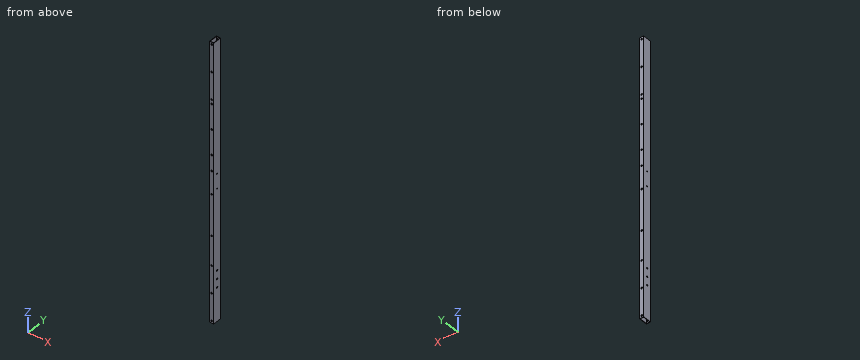
from build123d import *

# Parameters (mm, degrees)
SKETCH_1_W          = 10
SKETCH_1_H          = 20
SKETCH_1_W_2        = 7.6
SKETCH_1_H_2        = 17.6
EXTRUDE_1_DEPTH     = 660
SKETCH_2_R          = 2
CUT_EXTRUDE_1_DEPTH = 661.321891202
SKETCH_3_R          = 1.5
SKETCH_3_R_2        = 2
CUT_EXTRUDE_2_DEPTH = 661.151497764


with BuildPart() as part:
    # ｽｹｯﾁ1 → 押し出し-薄板1 (new body)
    with BuildSketch(Plane.XY):
        Rectangle(SKETCH_1_W, SKETCH_1_H)
        Rectangle(SKETCH_1_W_2, SKETCH_1_H_2, mode=Mode.SUBTRACT)
    extrude(amount=EXTRUDE_1_DEPTH)

    # ｽｹｯﾁ2 → ｶｯﾄ - 押し出し1 (cut, through all)
    with BuildSketch(Plane(origin=(0, 10, 0), x_dir=(1, 0, 0), z_dir=(0, 1, 0))):
        with Locations(Location((0, -525, 0), (0, 0, 270))):
            Circle(SKETCH_2_R)
        with Locations(Location((0, -655, 0), (0, 0, 270))):
            Circle(SKETCH_2_R)
        with Locations(Location((0, -590, 0), (0, 0, 270))):
            Circle(SKETCH_2_R)
        with Locations(Location((0, -5, 0), (0, 0, 270))):
            Circle(SKETCH_2_R)
        with Locations(Location((0, -70, 0), (0, 0, 270))):
            Circle(SKETCH_2_R)
        with Locations(Location((0, -135, 0), (0, 0, 270))):
            Circle(SKETCH_2_R)
        with Locations(Location((0, -515, 0), (0, 0, 270))):
            Circle(SKETCH_2_R)
        with Locations(Location((0, -357.5, 0), (0, 0, 270))):
            Circle(SKETCH_2_R)
        with Locations(Location((0, -302.5, 0), (0, 0, 270))):
            Circle(SKETCH_2_R)
        with Locations(Location((0, -395, 0), (0, 0, 270))):
            Circle(SKETCH_2_R)
        with Locations(Location((0, -455, 0), (0, 0, 270))):
            Circle(SKETCH_2_R)
        with Locations(Location((0, -205, 0), (0, 0, 270))):
            Circle(SKETCH_2_R)
    extrude(amount=-CUT_EXTRUDE_1_DEPTH, mode=Mode.SUBTRACT)

    # ｽｹｯﾁ3 → ｶｯﾄ - 押し出し2 (cut, through all)
    with BuildSketch(Plane(origin=(5, 0, 0), x_dir=(0, 0, -1), z_dir=(1, 0, 0))):
        with Locations(Location((-312.5, 0, 0), (0, 0, 90))):
            Circle(SKETCH_3_R)
        with Locations(Location((-347.5, 0, 0), (0, 0, 90))):
            Circle(SKETCH_3_R)
        with Locations(Location((-100, 0, 0), (0, 0, 90))):
            Circle(SKETCH_3_R_2)
        with Locations(Location((-80, 0, 0), (0, 0, 90))):
            Circle(SKETCH_3_R_2)
        with Locations(Location((-120, 0, 0), (0, 0, 90))):
            Circle(SKETCH_3_R_2)
    extrude(amount=-CUT_EXTRUDE_2_DEPTH, mode=Mode.SUBTRACT)


solid = part.part
Build history of the part. All positions in model axes, mm. Round coordinates to 2 decimals unless told otherwise and drop trailing zeros. Write each loop counter-clockwise with the first axis right and the second up, starting at its lowest first coordinate (ties: lowest second). Pieces come first, ordered by that corner, then holes. Notation, with made-up numbers: (82.25, -35) - (101.25, -35) arc R7 cw to (101.25, -31) - close; hole circle Ø3 at (38, -18). An arc over 180 degrees is marked (long way). Use CSV: the item, a comma, the result in double quotes.
(1) Wall check: line 1 (Y direction, x = -2.25, z = 356.5); line 2 (X direction, y = -4, z = 441.5); line 3 (X direction, y = -9.05, z = 205). Give the ranges that are in metal, low to high.
Response:
line 1,"-10 to -8.8, 8.8 to 10"
line 2,"-5 to -3.8, 3.8 to 5"
line 3,"-5 to -2, 2 to 5"
(2) Pin check, flat tips, straight feed: P1, Ø2.5, axis at y = 0, z = 312.5, coming from the +X side; P2, Ø5, axis at x = 0, z = 302.5, coming from the +Y side. Stop position of each tip, or through.
Response:
P1,"through"
P2,"y = 10"
(3) Band-saw the part on A-A (z = 142.5). Write the cut outline in (x, y).
Response:
outline,"(-5, -10) - (5, -10) - (5, 10) - (-5, 10) - close; hole (-3.8, -8.8) - (3.8, -8.8) - (3.8, 8.8) - (-3.8, 8.8) - close"
